Read the model definition and answer for the solid it produces. Units are mm, in the model's axes. A direction names the side the tool comes from. Coordinates: 2 decimals unless noted, no trailing zeros. Loops run counter-clockwise (first coordinate to the right, second up) from the corner with the lowest first, then second, coordinate; pieces in that order, holes last. Notation, with made-up numbers: (76.25, 36.25) -> (133.25, 36.25) arc R7 ccw to (133.25, 47.25) -> close; hole circle Ø7 at (44, 64). An arc over 180 degrees is marked (long way). Answer as CSV lines item,"result".
```python
from build123d import *

# Parameters (mm, degrees)
EXTRUDE_1_DEPTH     = 5
SKETCH_3_R          = 0.515
SKETCH_3_R_2        = 1
SKETCH_3_R_3        = 2.345
CUT_EXTRUDE_1_DEPTH = 6
EXTRUDE_2_DEPTH     = 3
CUT_EXTRUDE_2_DEPTH = 10


with BuildPart() as part:
    # 스케치1 → 보스-돌출1 (new body, symmetric)
    with BuildSketch(Plane(origin=(0, 0, 0), x_dir=(1, 0, 0), z_dir=(0, 1, 0))):
        with BuildLine():
            Line((-100, 5), (100, 5))
            ThreePointArc((100, 5), (105, 0), (100, -5))
            Line((100, -5), (-100, -5))
            ThreePointArc((-100, -5), (-105, 0), (-100, 5))
        make_face()
    extrude(amount=EXTRUDE_1_DEPTH, both=True)

    # 스케치3 → 컷-돌출1 (cut)
    with BuildSketch(Plane.XZ.offset(5)):
        with Locations((-90, 0)):
            Circle(SKETCH_3_R)
        with Locations((-88.036, 0)):
            Circle(SKETCH_3_R_2)
        with Locations((-86.072, 0)):
            Circle(SKETCH_3_R)
        with Locations((-84.108, 0)):
            Circle(SKETCH_3_R_2)
        with Locations((-82.144, 0)):
            Circle(SKETCH_3_R)
        with Locations((-80.18, 0)):
            Circle(SKETCH_3_R)
        with Locations((-75.93, 0)):
            Circle(SKETCH_3_R_3)
        with Locations((-71.68, 0)):
            Circle(SKETCH_3_R)
        with Locations((-69.716, 0)):
            Circle(SKETCH_3_R)
        with Locations((-67.752, 0)):
            Circle(SKETCH_3_R_2)
        with Locations((-65.788, 0)):
            Circle(SKETCH_3_R)
        with Locations((-61.86, 0)):
            Circle(SKETCH_3_R)
        with Locations((-63.824, 0)):
            Circle(SKETCH_3_R_2)
    extrude(amount=-CUT_EXTRUDE_1_DEPTH, mode=Mode.SUBTRACT)

    # 스케치5 → 보스-돌출2 (add)
    with BuildSketch(Plane.XZ.offset(5)):
        with BuildLine():
            Line((100, -5), (-35, -5))
            ThreePointArc((-35, -5), (-40, 0), (-35, 5))
            Line((-35, 5), (100, 5))
            ThreePointArc((100, 5), (105, 0), (100, -5))
        make_face()
    extrude(amount=EXTRUDE_2_DEPTH)

    # 스케치6 → 컷-돌출2 (cut)
    with BuildSketch(Plane.XZ.offset(8)):
        with BuildLine():
            Line((-35, 3), (100, 3))
            ThreePointArc((100, 3), (103, 0), (100, -3))
            Line((100, -3), (-35, -3))
            ThreePointArc((-35, -3), (-38, 0), (-35, 3))
        make_face()
    extrude(amount=-CUT_EXTRUDE_2_DEPTH, mode=Mode.SUBTRACT)


solid = part.part
```
Q1. For a pull along X with two mould halves and no side action, classify faces 1 (the face through (33, -3, -3)), 2 (the face through (105, -1, 0)), 3 (the face through (1, -1, -5)), 4 (the face through (-40, -6, 0)) as pulls with the +X half, pulls with the -X half, needs draft (parallel to the pull), parting line crosses it, or undercut.
Results:
face 1,"undercut"
face 2,"pulls with the +X half"
face 3,"needs draft"
face 4,"pulls with the -X half"
Q2. For faces 5 (the face through (103, -3, 0)), 6 (the face through (1, 5, 0)), determine the directions among +Z, -Z, +X, -X, +Y, -Y from which every point of the face is accessible in a straight line to the end or side of a thin tool.
Results:
face 5,"-Y"
face 6,"+Z, -Z, +X, -X, +Y"
Q3. Find the intervals of material crossed by probe 1 along Z at (x, y) = (84.5, 1.25); probe 2 along X at (y, z) = (-5.5, -4); probe 3 along Y at (x, z) = (-91, -2.5), in increasing order. Write a range as [from, to].
Results:
probe 1,"z = [-5, -3], [3, 5]"
probe 2,"x = [-38, 103]"
probe 3,"y = [-5, 5]"
Q4. A cutting plane is placed at A-A, the plane y = -2. Give the number of separate pieces and of enclosed holes in the cut face, and give its area (3 significant figures).
Results:
separate pieces,"1"
enclosed holes,"14"
area,"1,200 mm²"
Q5. Given pin 1 Ø2 at (y, z) = (2, 2.5) entering from -X; pin 2 Ø0.6 at (x, z) = (-80.18, 0) entering from -Y; pin 3 Ø1.6 at (x, z) = (-82.144, 0) entering from -Y, each flat-ended and moving along its own axis, determine where each tip first touches the part or whether it passes through.
Results:
pin 1,"stops at x = -104.77"
pin 2,"stops at y = 1"
pin 3,"stops at y = -5"
Q6. A cutting plane is placed at B-B, the plane x = 83. Write down the section's boundary in (y, z).
Results:
outline,"(-8, -5) -> (5, -5) -> (5, 5) -> (-8, 5) -> (-8, 3) -> (2, 3) -> (2, -3) -> (-8, -3) -> close"
